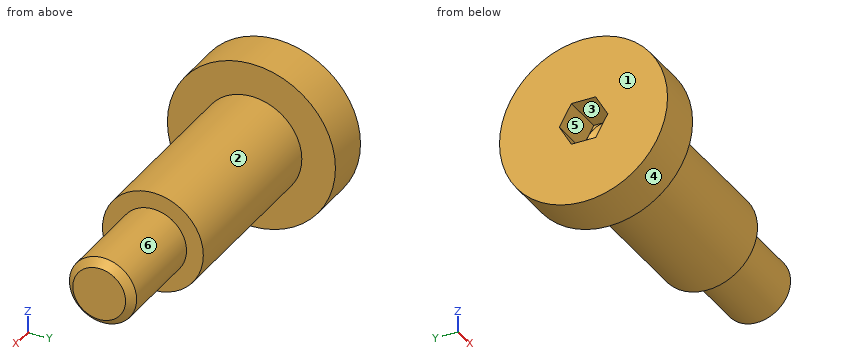
Autodesk Inventor part; units mm, degrees
ref_plane "YZ Plane" through (0, 0, 0) normal (1, 0, 0) x (0, 1, 0)
ref_plane "XZ Plane" through (0, 0, 0) normal (0, 1, 0) x (-1, 0, 0)
ref_plane "XY Plane" through (0, 0, 0) normal (0, 0, 1) x (1, 0, 0)
sketch "Sketch_1" plane through (0, 0, 0) normal (0, 0, 1) x (1, 0, 0)
  line L0 (11, 0) -> (-2.8, 0)
  line L1 (-2.8, 0) -> (-2.8, 5)
  line L2 (-2.8, 5) -> (0, 5)
  line L3 (0, 5) -> (0, 3)
  line L4 (0, 3) -> (11, 3)
  line L5 (11, 3) -> (11, 0)
  line L6 (11, 0) -> (-2.8, 0)
revolve "Revolution1" add sketch "Sketch_1" angle 360 about axis through (11, 0, 0) along (1, 0, 0)
sketch "Sketch2" plane through (-2.8, 0, 0) normal (-1, 0, 0) x (0, 0, 1)
  point P0 (0, 0)
hole "Hole1" at (-2.8, 0, 0) direction (1, 0, 0) diameter 2.5 depth 2.5 tip angle 120
sketch "Sketch_3" plane through (-2.8, 0, 0) normal (1, 0, 0) x (0, 0, -1)
  line L0 (-1.25, -0.7217) -> (0, -1.4434)
  line L1 (0, -1.4434) -> (1.25, -0.7217)
  line L2 (1.25, -0.7217) -> (1.25, 0.7217)
  line L3 (1.25, 0.7217) -> (0, 1.4434)
  line L4 (0, 1.4434) -> (-1.25, 0.7217)
  line L5 (-1.25, 0.7217) -> (-1.25, -0.7217)
extrude "Extrusion1" cut sketch "Sketch_3" along normal blind 2.5
sketch "Sketch_6" plane through (0, 0, 0) normal (0, 0, 1) x (1, 0, 0)
  line L0 (17, 0) -> (11, 0)
  line L1 (11, 0) -> (11, 2)
  line L2 (11, 2) -> (16.5705, 2)
  line L3 (16.5705, 2) -> (17, 1.5705)
  line L4 (17, 1.5705) -> (17, 0)
  line L5 (17, 0) -> (11, 0)
revolve "Revolution2" add sketch "Sketch_6" angle 360 about axis through (17, 0, 0) along (1, 0, 0)
thread "Thread1"
properties part number "DBTS4-11-6"
The listing builds one solid part. Answer for the finished solid, in the listing's coordinates (mm). Face numbers are marked on the shaded views. A direction names the side the tool comes from. Coordinates: 2 decimals unless noted, no trailing zeros. Order: outer loops, then holes, each group sorted by start corner. A loop starts at its lowest first (then second) coordinate and runs counter-clockwise, first axis right, second up. Notation, with made-up numbers: (-3, 8.5) -> (56, 8.5) arc R19 cw to (56, 37.5) -> close; hole circle Ø8 at (-32, -23.5). An arc over 180 degrees is marked (long way). Answer in a Markdown table with one row per item. Add a question column.
Item 1: Find section C-C (x = 11.25). Write down the section's boundary in (y, z).
Item 2: Find section A-A (x = 5.75). Write down the section's boundary in (y, z).
Item 3: Find the intervals of material crossed by L1, parallel to X at y = -1.75, z = 1.25; L2, parallel to Z at x = 6, y = 0; L3, parallel to X at y = 2.5, z = 3.75, in increasing order. Write a range as from..to.
Item 4: Find section B-B (z = 3.5). Write down the section's boundary in (x, y).
Item 5: Each of these flat-tipped pins is pushed along its axis until it touches: P1, Ø3, axis at y = -1.5, z = -2, coming from the +X side; P2, Ø3, axis at x = 14, z = 1.5, coming from the +Y side; P3, Ø6, axis at x = 8, z = -3.5, coming from the +Y side; P4, Ø4, axis at x = 8, y = -3.5, coming from the +Z side. Where does it stop, or does it pass through?
Item 6: Which of the six approach directions +Z, -Z, +X, -X, +Y, -Y give full straight-line access (tool end or side, diameter ignored) to the marked faces 4, 5 and 6?
Item 7: Determine the mould class of the marked faces 1, 2 and 3 for opening direction Y: +Y half, -Y half, draft (parallel to the pull), parting line (faces both ways), or undercut.
Result set:
| question | item | result |
|---|---|---|
| 1 | outline | circle Ø4 at (0, 0) |
| 2 | outline | circle Ø6 at (0, 0) |
| 3 | L1 | x = -2.8..11 |
| 3 | L2 | z = -3..3 |
| 3 | L3 | x = -2.8..0 |
| 4 | outline | (-2.8, -3.57) -> (0, -3.57) -> (0, 3.57) -> (-2.8, 3.57) -> close |
| 5 | P1 | stops at x = 17 |
| 5 | P2 | stops at y = 2 |
| 5 | P3 | stops at y = 2.96 |
| 5 | P4 | stops at z = 2.6 |
| 6 | face 4 | +X, -X |
| 6 | face 5 | -X |
| 6 | face 6 | +X |
| 7 | face 1 | draft |
| 7 | face 2 | parting line |
| 7 | face 3 | undercut |
